```python
from build123d import *

# Parameters (mm, degrees)
F1_DEPTH  = 3.175
F2_R      = 1.27
F1_FACE_W = 3.302
F1_FACE_H = 3.175
F3_DEPTH  = 1.143


with BuildPart() as f1:
    # F0 (on Top) → F1 (new body)
    with BuildSketch(Plane.XY):
        with BuildLine():
            Line((23.828722, -50.8), (30.178722, -50.8))
            ThreePointArc((30.178722, -50.8), (31.301254, -50.335032), (31.766222, -49.2125))
            Line((31.766222, -49.2125), (31.766222, 49.2125))
            ThreePointArc((31.766222, 49.2125), (31.301254, 50.335032), (30.178722, 50.8))
            Line((30.178722, 50.8), (17.241719, 50.8))
            ThreePointArc((17.241719, 50.8), (16.209511, 50.41861), (15.673269, 49.457696))
            Line((15.673269, 49.457696), (3.169756, -30.523921))
            Line((3.169756, -30.523921), (2.188974, -36.797721))
            Line((2.188974, -36.797721), (-4.084826, -35.816939))
            Line((-4.084826, -35.816939), (-9.982198, -34.895004))
            ThreePointArc((-9.982198, -34.895004), (-14.13118, -32.363933), (-15.275216, -27.640422))
            Line((-15.275216, -27.640422), (-14.294434, -21.366622))
            ThreePointArc((-14.294434, -21.366622), (-19.610562, -14.114872), (-26.862312, -19.431))
            Line((-26.862312, -19.431), (-31.479717, -48.967304))
            ThreePointArc((-31.479717, -48.967304), (-31.117378, -50.244708), (-29.911267, -50.8))
            Line((-29.911267, -50.8), (-23.053267, -50.8))
            Line((-23.053267, -50.8), (-23.053267, -41.148))
            Line((-23.053267, -41.148), (-19.751267, -41.148))
            Line((-19.751267, -41.148), (-19.751267, -50.8))
            Line((-19.751267, -50.8), (0, -50.8))
            Line((0, -50.8), (20.526722, -50.8))
            Line((20.526722, -50.8), (20.526722, -24.13))
            Line((20.526722, -24.13), (23.828722, -24.13))
            Line((23.828722, -24.13), (23.828722, -50.8))
        make_face()
        with BuildLine():
            Line((2.188974, -36.797721), (3.169756, -30.523921))
            ThreePointArc((3.169756, -30.523921), (0.638685, -34.672903), (-4.084826, -35.816939))
            Line((-4.084826, -35.816939), (2.188974, -36.797721))
        make_face()
    extrude(amount=F1_DEPTH)

    # F2
    f2_edges = [f1.edges().sort_by_distance(p)[0] for p in [
        (23.828722, -50.8, 1.5875),
        (-19.751267, -50.8, 1.5875),
        (20.526722, -50.8, 1.5875),
        (-23.053267, -50.8, 1.5875),
    ]]
    fillet(f2_edges, radius=F2_R)

    # F1_face (on face) → F3 (cut)
    with BuildSketch(Plane(origin=(-21.402267, -41.148, 1.5875), x_dir=(1, 0, 0), z_dir=(0, -1, 0))):
        Rectangle(F1_FACE_W, F1_FACE_H)
    extrude(amount=-F3_DEPTH, mode=Mode.SUBTRACT)


solid = f1.part
```
Part model, mm, in its own coordinate system. A direction names the side the tool comes from. Round coordinates to 2 decimals unless told otherwise and drop trailing zeros. Write each loop counter-clockwise with the first axis right and the second up, starting at its lowest first coordinate (ties: lowest second). Pieces come first, ordered by that corner, then holes. Notation, with made-up numbers: M 27.25,31 L 86.25,31 A33 cw 86.25,67 Z; hole C 44,42.5 d8. An arc over 180 degrees is marked long. One line per question, with ' | ' between items.
(1) Probe line 1 along X through (y, z) = (-30, 2.1); line 2 along X through (y, z) = (-21, 1.3); line 3 along Y through (x, z) = (-3.5, 0.85). List the from-to ranges inside material, lowest first.
Answer key:
line 1: x = -28.51 to -15.2, 3.25 to 20.53, 23.83 to 31.77 | line 2: x = -27.11 to -14.25, 4.66 to 31.77 | line 3: y = -50.8 to -35.88
(2) Pin check, flat tips, straight feed: pin 1 (10 mm diameter, centred on x = -21, y = -28, fed in from -Z); pin 2 (1 mm diameter, centred on y = -31.5, z = 2, fed in from -X); pin 3 (1.6 mm diameter, centred on x = -22, z = 1.5, fed in from -Y) (3 decimals); pin 4 (1.6 mm diameter, centred on y = -46, z = 2, fed in from -X). Stop position of each tip, or through.
Answer key:
pin 1: stops at z = 0 | pin 2: stops at x = -28.83 | pin 3: stops at y = -40.005 | pin 4: stops at x = -31.14
(3) Saw through at B-B on x = -7.5. Write the cut outline in (y, z) (3 decimals), then the cut area to 3 significant figures.
Answer key:
outline: M -50.8,0 L -35.283,0 L -35.283,3.175 L -50.8,3.175 Z | area: 49.3 mm^2
(4) Saw through at C-C on y = 4. Write the cut outline in (x, z) (3 decimals), then the cut area to 3 significant figures.
Answer key:
outline: M 8.567,0 L 31.766,0 L 31.766,3.175 L 8.567,3.175 Z | area: 73.7 mm^2
(5) 3-axis set-ups, long thin cutter, end or side, ignore diameter. For faces 5 (the face through (28, -50.8, 2)), 6 (the face through (-29.14, -33.99, 1.57)), 7 (the face through (-6.992, -35.362, 1.565)), 8 (the face through (-14.792, -24.547, 1.565)), 9 (the face through (23.829, -37, 2)): which of +Z, -Z, +X, -X, +Y, -Y reach the whole face in a straight line?
Answer key:
face 5: +Z, -Z, +X, -X, -Y | face 6: +Z, -Z, -X, +Y | face 7: +Z, -Z, +Y | face 8: +Z, -Z | face 9: +Z, -Z, -Y
(6) Two-plate mould, pull along Y, no slides. Class faces 1 (the face through (-14.09, -32.42, 1.57)), 2 (the face through (-19.751, -45, 2)), 3 (the face through (9.51, 10.03, 1.57)), 4 (the face through (22, -24.13, 2)): released by +Y, released by -Y, zero draft, split by the parting line, or undercut.
Answer key:
face 1: undercut | face 2: zero draft | face 3: released by +Y | face 4: released by -Y
